Source: CAD feature listing. Evaluate the final solid. Frame: model axes, mm. A direction names the side the tool comes from. Round coordinates to 2 decimals unless told otherwise and drop trailing zeros. Loops run counter-clockwise (first coordinate to the right, second up) from the corner with the lowest first, then second, coordinate; pieces in that order, holes last. Notation, with made-up numbers: M -30,-29.75 L -10,-29.75 A19 cw -10,-21.75 Z; hole C 15,56 d1. An arc over 180 degrees is marked long. Answer as CSV lines item,"result". Start each with the question number.
```python
from build123d import *

# Parameters (mm, degrees)
SKETCH1_W           = 20
SKETCH1_H           = 12
SKETCH1_R           = 1.75
BOSS_EXTRUDE1_DEPTH = 5
SKETCH2_W           = 3
SKETCH2_H           = 12
BOSS_EXTRUDE2_DEPTH = 0.6
SKETCH3_R           = 3
CUT_EXTRUDE1_DEPTH  = 3


with BuildPart() as part:
    # Sketch1 → Boss-Extrude1 (new body)
    with BuildSketch(Plane.XY):
        with Locations((10, 6)):
            Rectangle(SKETCH1_W, SKETCH1_H)
        with Locations((10, 6)):
            Circle(SKETCH1_R, mode=Mode.SUBTRACT)
    extrude(amount=BOSS_EXTRUDE1_DEPTH)

    # Sketch2 → Boss-Extrude2 (add)
    with BuildSketch(Plane.XY.offset(5)):
        with Locations((1.5, 6)):
            Rectangle(SKETCH2_W, SKETCH2_H)
    extrude(amount=BOSS_EXTRUDE2_DEPTH)

    # Sketch3 → Cut-Extrude1 (cut)
    with BuildSketch(Plane(origin=(0, 0, 0), x_dir=(-1, 0, 0), z_dir=(0, 0, -1))):
        with Locations((-10, 6)):
            Circle(SKETCH3_R)
    extrude(amount=-CUT_EXTRUDE1_DEPTH, mode=Mode.SUBTRACT)


solid = part.part
```
1) Section C-C, the plane z = 1.35. Return loops of the section in (x, y), and give its area (3 significant figures).
2) Section D-D, the plane y = 2. Return loops of the section in (x, z).
3) Mould query, pull axis X, two halves, no side actions, for faces 4 (the flat face through (12, 9, 0)), 5 (the flat face through (20, 6, 2)), 6 (the flat face through (8, 6, 3)). Classes: pulls with the +X half, pulls with the -X half, needs draft (parallel to the pull), parting line crosses it, or undercut.
4) Ray query, line 1 along Y through (x, z) = (10, 4.3); line 2 along Y through (x, z) = (10, 1.85); line 3 along X through (y, z) = (6, 4.25). Return the intervals inside material, ascending.
5) Contact query for flat-ended pins moving along their axis: pin 1 Ø6 at (x, y) = (9.5, 3.5) entering from +Z; pin 2 Ø0.7 at (y, z) = (5, 5.5) entering from +X. Output: stop coordinate, or through.
6) Section B-B, the plane x = 10. Return loops of the section in (y, z), and give its area (3 significant figures).
7) Section A-A, the plane y = 6. Return loops of the section in (x, z).
8) Access query for faces 1 (the flat face through (11.4, 7.4, 5)), 2 (the flat face through (10, 12, 3)), 3 (the cylindrical face through (12.4, 4.2, 1.5)). Directions: +Z, -Z, +X, -X, +Y, -Y. A direction counts if a zero-diameter tool reaches every point of the face in a straight line with its end or side. Return the directions, or none.
Findings below:
1,outline,"M 0,0 L 20,0 L 20,12 L 0,12 Z; hole C 10,6 d6"
1,area,"212 mm²"
2,outline,"M 0,0 L 20,0 L 20,5 L 3,5 L 3,5.6 L 0,5.6 Z"
3,face 4,"needs draft"
3,face 5,"pulls with the +X half"
3,face 6,"undercut"
4,line 1,"0 to 4.25, 7.75 to 12"
4,line 2,"0 to 3, 9 to 12"
4,line 3,"0 to 8.25, 11.75 to 20"
5,pin 1,"z = 5"
5,pin 2,"x = 3"
6,outline,"M 0,0 L 3,0 L 3,3 L 4.25,3 L 4.25,5 L 0,5 Z; M 7.75,3 L 9,3 L 9,0 L 12,0 L 12,5 L 7.75,5 Z"
6,area,"35.0 mm²"
7,outline,"M 0,0 L 7,0 L 7,3 L 8.25,3 L 8.25,5 L 3,5 L 3,5.6 L 0,5.6 Z; M 11.75,3 L 13,3 L 13,0 L 20,0 L 20,5 L 11.75,5 Z"
8,face 1,"+Z, +X, +Y, -Y"
8,face 2,"+Z, -Z, +X, -X, +Y"
8,face 3,"-Z"
